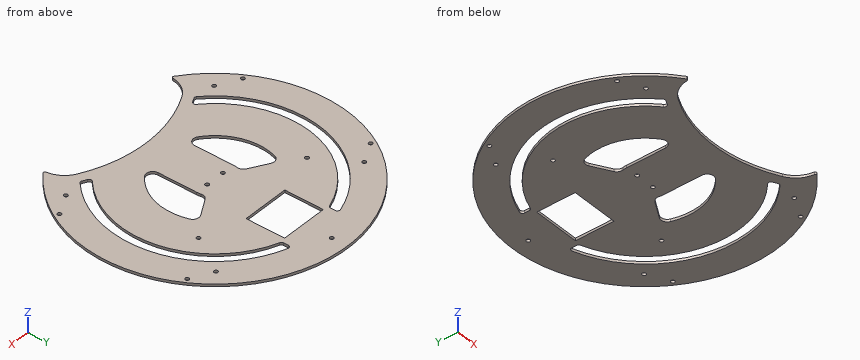
Autodesk Inventor part; units mm, degrees
ref_plane "YZ Plane" through (0, 0, 0) normal (1, 0, 0) x (0, 1, 0)
ref_plane "XZ Plane" through (0, 0, 0) normal (0, 1, 0) x (-1, 0, 0)
ref_plane "XY Plane" through (0, 0, 0) normal (0, 0, 1) x (1, 0, 0)
sketch "Sketch1" plane through (0, 0, 0) normal (0, 0, 1) x (1, 0, 0)
  line L0 (18.5032, 45.3912) -> (18.5032, 14.8912)
  line L1 (18.5032, 14.8912) -> (-18.4968, 14.8912)
  line L2 (-18.4968, 14.8912) -> (-18.4968, 45.3912)
  line L3 (-18.4968, 45.3912) -> (18.5032, 45.3912)
  arc A0 (17.5017, -55.6702) -> (25.4619, -59.6998) centre (22.5017, -55.6702) ccw
  line L4 (17.5017, -55.6702) -> (17.5016, -25.0441)
  arc A1 (17.5016, -25.0441) -> (17.2066, -21.8442) centre (0.0033, -25.0441) ccw
  arc A2 (19.6222, -16.5997) -> (17.2066, -21.8442) centre (22.1222, -20.9298) ccw
  line L5 (19.6222, -16.5997) -> (33.5153, -8.5785)
  arc A3 (40.7535, -11.3119) -> (33.5153, -8.5785) centre (36.0153, -12.9086) ccw
  arc A4 (25.4619, -59.6998) -> (40.7535, -11.3119) centre (0.0033, -25.0441) ccw
  arc A5 (-17.2054, -21.8447) -> (-19.6211, -16.6006) centre (-22.1212, -20.9307) ccw
  arc A6 (-17.2054, -21.8447) -> (-17.5003, -25.0442) centre (0.0033, -25.0441) ccw
  line L6 (-17.5003, -25.0442) -> (-17.5003, -55.6665)
  arc A7 (-25.4611, -59.6955) -> (-17.5003, -55.6665) centre (-22.5003, -55.6665) ccw
  arc A8 (-40.7482, -11.3157) -> (-25.4611, -59.6955) centre (0.0033, -25.0441) ccw
  arc A9 (-33.5098, -8.5818) -> (-40.7482, -11.3157) centre (-36.0099, -12.9119) ccw
  line L7 (-33.5098, -8.5818) -> (-19.6211, -16.6006)
  line L8 (22.5032, 47.8371) -> (22.5032, 51.6387)
  arc A10 (25.1118, 53.5439) -> (22.5032, 51.6387) centre (24.5032, 51.6387) ccw
  arc A11 (-25.1056, 53.5343) -> (-69.0178, 20.1345) centre (0.0033, -25.0441) ccw
  arc A12 (-22.4968, 51.6291) -> (-25.1056, 53.5343) centre (-24.4968, 51.6291) ccw
  line L9 (-22.4968, 51.6291) -> (-22.4968, 47.8394)
  arc A13 (53.5122, -86.077) -> (55.8167, -85.7905) centre (54.4635, -84.3178) ccw
  arc A14 (53.5122, -86.077) -> (50.1516, -84.3322) centre (-0.0002, -185.037) ccw
  arc A15 (-50.1523, -84.3319) -> (-53.5093, -86.0748) centre (-0.0002, -185.037) ccw
  arc A16 (-55.8138, -85.7882) -> (-53.5093, -86.0748) centre (-54.4606, -84.3155) ccw
  arc A17 (-62.339, -109.5339) -> (-60.7504, -108.8306) centre (-61.7453, -108.7292) ccw
  arc A18 (-50.0022, -92.7062) -> (-60.7504, -108.8306) centre (-40.1313, -110.9304) ccw
  arc A19 (50.001, -92.7085) -> (-50.0022, -92.7062) centre (-0.0027, -185.0388) ccw
  arc A20 (60.7494, -108.8311) -> (50.001, -92.7085) centre (40.1315, -110.9322) ccw
  arc A21 (60.7494, -108.8311) -> (62.3379, -109.5344) centre (61.7442, -108.7297) ccw
  arc A22 (62.3379, -109.5344) -> (-62.339, -109.5339) centre (-0.0002, -25.0416) ccw
  arc A23 (49.7154, -81.0462) -> (23.8658, 45.9414) centre (-0.0002, -25.0416) ccw
  arc A24 (-23.8596, 45.9436) -> (-49.7161, -81.046) centre (-0.0002, -25.0416) ccw
  arc A25 (55.661, -85.9197) -> (24.8977, 53.5994) centre (-0.0002, -25.0416) ccw
  arc A26 (-25.052, 53.5506) -> (-55.6938, -85.89) centre (-0.0002, -25.0416) ccw
  arc A27 (-50.1523, -84.3319) -> (-49.7161, -81.046) centre (-51.0439, -82.5417) ccw
  arc A28 (49.7154, -81.0462) -> (50.1516, -84.3322) centre (51.0431, -82.5419) ccw
  arc A29 (22.5032, 47.8371) -> (23.8658, 45.9414) centre (24.5032, 47.8371) ccw
  arc A30 (-23.8596, 45.9436) -> (-22.4968, 47.8394) centre (-24.4968, 47.8394) ccw
  point P0 (0, 0)
  point P1 (22.5032, 46.385)
  point P2 (-22.4968, 46.3872)
  dimension "d31" = 2
extrude "Extrusion11" add sketch "Sketch1" along normal blind 2
ref_plane "Work Plane9" through (0, 0, 2) normal (0, 0, 1) x (1, 0, 0)
sketch "Sketch4" plane through (0, 0, 2) normal (0, 0, 1) x (1, 0, 0)
  circle A0 centre (0.0001, -25.0412) radius 10.8
  line L0 (0.0001, -25.0412) -> (-7.4999, -25.0412) construction
  circle A1 centre (-7.4999, -25.0412) radius 1.5
  line L1 (0.0001, -25.0412) -> (7.5001, -25.0412) construction
  circle A2 centre (7.5001, -25.0412) radius 1.5
  point P0 (0, 0)
  dimension "d19" = 7.5
  dimension "d20" = 3
  dimension "d21" = 7.5
  dimension "d22" = 3
extrude "Extrusion7" cut sketch "Sketch4" against normal up to next contours A1 | A2
sketch "Sketch8" plane through (0, 0, 0) normal (0, 0, -1) x (-1, 0, 0)
  circle A0 centre (70.8591, 34.4165) radius 1.5
  circle A1 centre (87.6853, 25.5834) radius 1.5
  circle A2 centre (87.6853, -75.6666) radius 1.5
  circle A3 centre (70.8591, -84.4992) radius 1.5
  circle A4 centre (51.8178, 4.8745) radius 1.5
  circle A5 centre (0, 67.4586) radius 1.5
  circle A6 centre (-70.8591, 34.4165) radius 1.5
  circle A7 centre (-51.8178, 4.8745) radius 1.5
  circle A8 centre (-87.6849, 25.5834) radius 1.5
  circle A9 centre (-87.6849, -75.6666) radius 1.5
  circle A10 centre (-70.8591, -84.4992) radius 1.5
  point P0 (0, 0)
extrude "Extrusion12" cut sketch "Sketch8" against normal blind 2
properties part number "4th Board"
Source: CAD feature listing. Evaluate the final solid. Frame: model axes, mm. Coordinates: 2 decimals unless noted, no trailing zeros. Write each question's results on one line, items separated by ' | '. Start each with the question number.
Item 1: Cut plane A-A (z = 0.35). Count the separate pieces of the cut face and the enclosed holes in it, and give its area (3 significant figures).
Item 2: First-contact query: pin 1 Ø2.5 at (x, y) = (-7.5, -25.04) entering from +Z; pin 2 Ø0.6 at (x, z) = (-0.5, 1) entering from -Y; pin 3 Ø1 at (y, z) = (40.5, 0.5) entering from -X. Flat tips, straight axial feed; report the tip coordinate or a pass-through.
Item 3: Line query: probe 1 along Y at (x, z) = (30.5, 1.55); probe 2 along Y at (x, z) = (-66, 0.2); probe 3 along X at (y, z) = (-28, 0.95). Output: solid intervals per line, ascending.
Checked values:
1) separate pieces: 1 | enclosed holes: 18 | area: 24,300 mm2
2) pin 1: passes through | pin 2: stops at y = -80.04 | pin 3: stops at x = -82.43
3) probe 1: y = -84.57 to -55.36, -10.32 to 43.35, 51.6 to 75.43 | probe 2: y = -106.71 to -74.52, -60.43 to 10.34, 24.44 to 56.62 | probe 3: x = -104.96 to -82.44, -74.83 to -42.9, -17.5 to 17.5, 42.9 to 74.83, 82.43 to 104.96
